Here's how the part is built. I have some questions about the finished solid (model axes, mm). Face numbers are marked on the shaded views. A direction names the side the tool comes from. Give positions to 0.01 mm unless a question says otherwise; leave off trailing zeros. Write each loop counter-clockwise with the first axis right and the second up, starting at its lowest first coordinate (ties: lowest second). Pieces come first, ordered by that corner, then holes. Notation, with made-up numbers: (69.5, 35.5) -> (81.5, 35.5) arc R4 cw to (81.5, 39.5) -> close; hole circle Ø8 at (13, 51). An arc over 180 degrees is marked (long way). Put each result on its own line as item: value. Start each with the question number.
from build123d import *

# Parameters (mm, degrees)
SKETCH1_W                      = 59.9
SKETCH1_H                      = 34.76
BASE_FLANGE1_DEPTH             = 2
EDGE_FLANGE1_STRIP_W           = 10
EDGE_FLANGE1_STRIP_H           = 2
EDGE_FLANGE1_STRIP_CUT_DEPTH   = 34.76
EDGE_FLANGE1_STRIP_2_W         = 10
EDGE_FLANGE1_STRIP_2_H         = 2
EDGE_FLANGE1_STRIP_CUT_2_DEPTH = 34.76
EDGE_FLANGE1_DEPTH             = 34.76
EDGE_FLANGE1_BEND_DEPTH        = 34.76
FILLET1_R                      = 0.5
SKETCH8_R                      = 1.17
CUT_EXTRUDE1_DEPTH             = 10


# Sheet-metal steps are written as plain solids
with BuildPart() as part:
    # Sketch1 → Base-Flange1 (new body)
    with BuildSketch(Plane(origin=(0, 0, 0), x_dir=(1, 0, 0), z_dir=(0, 1, 0))):
        Rectangle(SKETCH1_W, SKETCH1_H)
    extrude(amount=-BASE_FLANGE1_DEPTH)

    # Edge-Flange1 strip (across the edge) → Edge-Flange1 strip cut (cut)
    with BuildSketch(Plane(origin=(-29.95, 0, -17.38), x_dir=(1, 0, 0), z_dir=(0, 0, 1))):
        with Locations((-2, -1)):
            Rectangle(EDGE_FLANGE1_STRIP_W, EDGE_FLANGE1_STRIP_H)
    extrude(amount=EDGE_FLANGE1_STRIP_CUT_DEPTH, mode=Mode.SUBTRACT)

    # Edge-Flange1 strip 2 (across the edge) → Edge-Flange1 strip cut 2 (cut)
    with BuildSketch(Plane(origin=(29.95, 0, 17.38), x_dir=(-1, 0, 0), z_dir=(0, 0, -1))):
        with Locations((-2, -1)):
            Rectangle(EDGE_FLANGE1_STRIP_2_W, EDGE_FLANGE1_STRIP_2_H)
    extrude(amount=EDGE_FLANGE1_STRIP_CUT_2_DEPTH, mode=Mode.SUBTRACT)

    # Edge-Flange1 section (across the edge) → Edge-Flange1 (add)
    with BuildSketch(Plane(origin=(-29.95, 0, -17.38), x_dir=(1, 0, 0), z_dir=(0, 0, 1))):
        with BuildLine():
            Line((0, 1), (0, 18))
            Line((0, 18), (2, 18))
            Line((2, 18), (2, 1))
            ThreePointArc((2, 1), (2.292893219, 0.292893219), (3, 0))
            Line((3, 0), (3, -2))
            ThreePointArc((3, -2), (0.878679656, -1.121320344), (0, 1))
        make_face()
    extrude(amount=EDGE_FLANGE1_DEPTH)

    # Edge-Flange1 section 2 (across the edge) → Edge-Flange1 bend (add)
    with BuildSketch(Plane(origin=(29.95, 0, 17.38), x_dir=(-1, 0, 0), z_dir=(0, 0, -1))):
        with BuildLine():
            Line((0, 1), (0, 18))
            Line((0, 18), (2, 18))
            Line((2, 18), (2, 1))
            ThreePointArc((2, 1), (2.292893219, 0.292893219), (3, 0))
            Line((3, 0), (3, -2))
            ThreePointArc((3, -2), (0.878679656, -1.121320344), (0, 1))
        make_face()
    extrude(amount=EDGE_FLANGE1_BEND_DEPTH)

    # Fillet1
    fillet1_edges = [part.edges().sort_by_distance(p)[0] for p in [
        (0, 0, 17.38),
        (0, 0, -17.38),
        (-27.657106781, 0.292893219, -17.38),
        (-27.657106781, 0.292893219, 17.38),
        (-27.95, 9.5, 17.38),
        (-27.95, 9.5, -17.38),
        (-29.95, 18, 0),
        (-27.95, 18, 0),
        (27.657106781, 0.292893219, 17.38),
        (27.657106781, 0.292893219, -17.38),
        (27.95, 9.5, 17.38),
        (27.95, 9.5, -17.38),
        (29.95, 18, 0),
        (27.95, 18, 0),
    ]]
    fillet(fillet1_edges, radius=FILLET1_R)

    # Sketch8 → Cut-Extrude1 (cut)
    with BuildSketch(Plane(origin=(0, 0, 0), x_dir=(1, 0, 0), z_dir=(0, 1, 0))):
        with Locations(Location((0, 0, 0), (0, 0, 270))):
            Circle(SKETCH8_R)
        with Locations(Location((0, 9, 0), (0, 0, 270))):
            Circle(SKETCH8_R)
        with Locations(Location((9, 0, 0), (0, 0, 270))):
            Circle(SKETCH8_R)
        with Locations(Location((0, -9, 0), (0, 0, 270))):
            Circle(SKETCH8_R)
        with Locations(Location((-9, 0, 0), (0, 0, 270))):
            Circle(SKETCH8_R)
    extrude(amount=-CUT_EXTRUDE1_DEPTH, mode=Mode.SUBTRACT)


solid = part.part
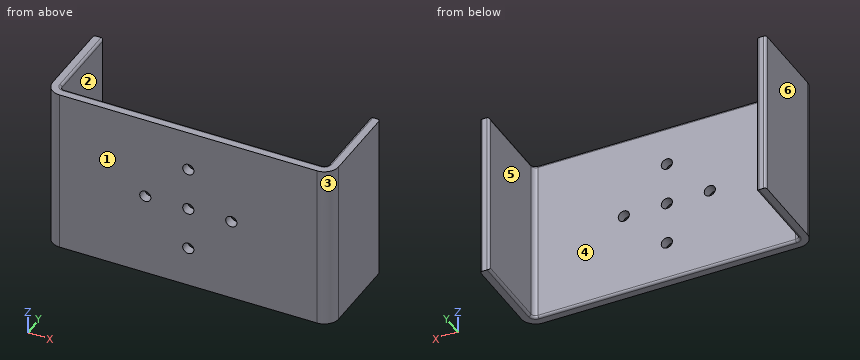
1) I want a section at B-B, the plane x = 0. Write out the boundary of the cut face in (y, z).
2) I need wall thicknesses on probe 1 along X at (y, z) = (1.25, -8); probe 2 along X at (y, z) = (-1.55, 0); probe 3 along Y at (x, z) = (27, -1.5). Which ranges of each line are inside material? Lowest first, please.
3) Thinking about a two-plate mould opening in X: for the marked faces 3, 4, 5 and 6, which applies, released by +X, released by -X, zero draft, split by the parting line, or undercut?
4) I want a section at D-D, the plane z = -9. Write out the boundary of the cut face in (x, y), and give its area (3 significant figures).
5) I'm going to push flat-ended pins straight in: pin 1 Ø8 at (x, y) = (-13.5, 7.5) entering from +Z; pin 2 Ø3 at (x, z) = (0, 9) entering from +Y; pin 3 Ø3 at (x, z) = (0, 0) entering from -Y. Where does each tip first touch, or does it pass through?
6) Which directions (+Z, -Z, +X, -X, +Y, -Y) give clear straight access to the entire face, cutting with the end or side of a thin tool? Please do the marked faces 1 and 2.
7) I want a section at C-C, the plane y = 10.75. Write out the boundary of the cut face in (x, z), and give its area (3 significant figures).
8) I want a section at A-A, the plane z = 0. Write out the boundary of the cut face in (x, y), and give its area (3 significant figures).
Established:
1. outline: (-2, -17.38) -> (-0.5, -17.38) arc R0.5 ccw to (0, -16.88) -> (0, -10.17) -> (-2, -10.17) -> close; (-2, -7.83) -> (0, -7.83) -> (0, -1.17) -> (-2, -1.17) -> close; (-2, 1.17) -> (0, 1.17) -> (0, 7.83) -> (-2, 7.83) -> close; (-2, 10.17) -> (0, 10.17) -> (0, 16.88) arc R0.5 ccw to (-0.5, 17.38) -> (-2, 17.38) -> close
2. probe 1: x = -29.95 to -27.95, 27.95 to 29.95
2. probe 2: x = -28.53 to -10.17, -7.83 to -1.17, 1.17 to 7.83, 10.17 to 28.53
2. probe 3: y = -2 to 0
3. face 3: released by +X
3. face 4: undercut
3. face 5: undercut
3. face 6: released by -X
4. outline: (-29.95, 1) arc R3 ccw to (-26.95, -2) -> (-1.17, -2) -> (-1.17, 0) -> (-26.95, 0) arc R1 cw to (-27.95, 1) -> (-27.95, 17.5) arc R0.5 ccw to (-28.45, 18) -> (-29.45, 18) arc R0.5 ccw to (-29.95, 17.5) -> close; (1.17, -2) -> (26.95, -2) arc R3 ccw to (29.95, 1) -> (29.95, 17.5) arc R0.5 ccw to (29.45, 18) -> (28.45, 18) arc R0.5 ccw to (27.95, 17.5) -> (27.95, 1) arc R1 cw to (26.95, 0) -> (1.17, 0) -> close
4. area: 183 mm2
5. pin 1: passes through
5. pin 2: stops at y = 0
5. pin 3: stops at y = -2
6. face 1: +Z, -Z, +X, -X, -Y
6. face 2: +Z, -Z, +Y
7. outline: (-29.95, -17.38) -> (-28.45, -17.38) arc R0.5 ccw to (-27.95, -16.88) -> (-27.95, 16.88) arc R0.5 ccw to (-28.45, 17.38) -> (-29.95, 17.38) -> close; (27.95, -16.88) arc R0.5 ccw to (28.45, -17.38) -> (29.95, -17.38) -> (29.95, 17.38) -> (28.45, 17.38) arc R0.5 ccw to (27.95, 16.88) -> close
7. area: 139 mm2
8. outline: (-29.95, 1) arc R3 ccw to (-26.95, -2) -> (-10.17, -2) -> (-10.17, 0) -> (-26.95, 0) arc R1 cw to (-27.95, 1) -> (-27.95, 17.5) arc R0.5 ccw to (-28.45, 18) -> (-29.45, 18) arc R0.5 ccw to (-29.95, 17.5) -> close; (-7.83, -2) -> (-1.17, -2) -> (-1.17, 0) -> (-7.83, 0) -> close; (1.17, -2) -> (7.83, -2) -> (7.83, 0) -> (1.17, 0) -> close; (10.17, -2) -> (26.95, -2) arc R3 ccw to (29.95, 1) -> (29.95, 17.5) arc R0.5 ccw to (29.45, 18) -> (28.45, 18) arc R0.5 ccw to (27.95, 17.5) -> (27.95, 1) arc R1 cw to (26.95, 0) -> (10.17, 0) -> close
8. area: 174 mm2
